from build123d import *

# Parameters (mm, degrees)
SKETCH1_R           = 10
BOSS_EXTRUDE1_DEPTH = 2.5
SKETCH5_W           = 1
SKETCH5_H           = 1
SKETCH6_W           = 1
SKETCH6_H           = 2
BOSS_EXTRUDE2_DEPTH = 0.5
SKETCH7_R           = 0.2
CUT_EXTRUDE1_DEPTH  = 1.5


with BuildPart() as part:
    # Sketch1 → Boss-Extrude1 (new body)
    with BuildSketch(Plane(origin=(0, 0, 0), x_dir=(0, 1, 0), z_dir=(0, 0, 1))):
        with Locations(Location((0, 0, 0), (0, 0, 270))):
            Circle(SKETCH1_R)
    extrude(amount=BOSS_EXTRUDE1_DEPTH)

    # Sketch5 → Cut-Revolve1 (revolve, cut)
    with BuildSketch(Plane(origin=(0, 0, 0), x_dir=(-1, 0, 0), z_dir=(0, 1, 0))):
        with Locations((-4.5, 2)):
            Rectangle(SKETCH5_W, SKETCH5_H)
        with Locations((-2.5, 2)):
            Rectangle(SKETCH5_W, SKETCH5_H)
        with Locations((-6.5, 2)):
            Rectangle(SKETCH5_W, SKETCH5_H)
        with Locations((-8.5, 2)):
            Rectangle(SKETCH5_W, SKETCH5_H)
    revolve(axis=Axis((0, 0, 2.5), (0, 0, -1)), mode=Mode.SUBTRACT)

    # Sketch6 → Boss-Extrude2 (add, symmetric)
    with BuildSketch(Plane(origin=(0, 0, 0), x_dir=(-1, 0, 0), z_dir=(0, 1, 0))):
        with Locations((-2.5, -1)):
            Rectangle(SKETCH6_W, SKETCH6_H)
        with Locations((-4.5, -1)):
            Rectangle(SKETCH6_W, SKETCH6_H)
        with Locations((-6.5, -1)):
            Rectangle(SKETCH6_W, SKETCH6_H)
        with Locations((-8.5, -1)):
            Rectangle(SKETCH6_W, SKETCH6_H)
    extrude(amount=BOSS_EXTRUDE2_DEPTH, both=True)

    # Sketch7 → Cut-Extrude1 (cut, symmetric)
    with BuildSketch(Plane(origin=(0, 0, 0), x_dir=(-1, 0, 0), z_dir=(0, 1, 0))):
        with Locations(Location((-8.5, -1.583373246, 0), (0, 0, 90))):
            Circle(SKETCH7_R)
        with Locations(Location((-6.5, -1.583373246, 0), (0, 0, 90))):
            Circle(SKETCH7_R)
        with Locations(Location((-4.5, -1.583373246, 0), (0, 0, 90))):
            Circle(SKETCH7_R)
        with Locations(Location((-2.5, -1.583373246, 0), (0, 0, 270))):
            Circle(SKETCH7_R)
    extrude(amount=CUT_EXTRUDE1_DEPTH, both=True, mode=Mode.SUBTRACT)


solid = part.part
Here's how the part is built. I have some questions about the finished solid (model axes, mm). A direction names the side the tool comes from. Coordinates: 2 decimals unless noted, no trailing zeros. Loops run counter-clockwise (first coordinate to the right, second up) from the corner with the lowest first, then second, coordinate; pieces in that order, holes last. Notation, with made-up numbers: (-21.5, 4.25) -> (29.5, 4.25) arc R20 cw to (29.5, 20.25) -> close; hole circle Ø7 at (-21, 24). An arc over 180 degrees is marked (long way). Use one line per item in the form item = value. Start each with the question number.
(1) On a 3-axis mill with a long thin cutter (end or side, diameter ignored), from which of +Z, -Z, +X, -X, +Y, -Y can I reach the whole of each face in a straight line? I mean faces 1 (the face through (5, 0, -1)), 2 (the face through (2, 0, -1)), 3 (the face through (2.5, -0.5, -1)). Say none if no direction works.
(2) If we section it at C-C (y = -4.25): Please give me the cut outline in (x, z), then the cut area to 3 significant figures.
(3) Will these pins go through, and if not, where does the flat tip stop? pin 1 (0.8 mm diameter, centred on y = 0, z = -1, fed in from +X); pin 2 (1.1 mm diameter, centred on x = 8.5, z = -1, fed in from +Y); pin 3 (6 mm diameter, centred on x = 4.5, y = 4.5, fed in from -Z).
(4) We'd pull the mould along X, two halves only. Please class faces 4 (the face through (4, 0, -1)), 5 (the face through (4.5, 0.5, -1)), 6 (the face through (9, 0, -1)): pulls with the +X half, pulls with the -X half, needs draft (parallel to the pull), parting line crosses it, or undercut.
(5) Please list where these lines run through material, in increasing order: line 1 along Z through (x, y) = (2.5, -0.15); line 2 along X through (y, z) = (0, -1.3); line 3 along Z through (x, y) = (-8, -1).
(6) If we section it at B-B (x = -5.75): Please give me the cut outline in (y, z).
(7) If we section it at A-A (z = -0.85): Please give me the cut outline in (x, y), then the cut area to 3 significant figures.
(8) If we section it at D-D (z = 0.25): Please give me the cut outline in (x, y), then the cut area to 3 significant figures.
Verdict:
q1.face_1 = -Z, +Y, -Y
q1.face_2 = -Z, -X, +Y, -Y
q1.face_3 = -Z, +X, -X, -Y
q2.outline = (-9.05, 0) -> (9.05, 0) -> (9.05, 2.5) -> (7.93, 2.5) -> (7.93, 1.5) -> (6.78, 1.5) -> (6.78, 2.5) -> (5.56, 2.5) -> (5.56, 1.5) -> (4.24, 1.5) -> (4.24, 2.5) -> (2.63, 2.5) -> (2.63, 1.5) -> (-2.63, 1.5) -> (-2.63, 2.5) -> (-4.24, 2.5) -> (-4.24, 1.5) -> (-5.56, 1.5) -> (-5.56, 2.5) -> (-6.78, 2.5) -> (-6.78, 1.5) -> (-7.93, 1.5) -> (-7.93, 2.5) -> (-9.05, 2.5) -> close
q2.area = 35.0 mm²
q3.pin_1 = 9
q3.pin_2 = 0.5
q3.pin_3 = 0
q4.face_4 = undercut
q4.face_5 = needs draft
q4.face_6 = pulls with the +X half
q5.line_1 = -2 to -1.78, -1.38 to 1.5
q5.line_2 = 2 to 3, 4 to 5, 6 to 7, 8 to 9
q5.line_3 = 0 to 1.5
q6.outline = (-8.18, 0) -> (8.18, 0) -> (8.18, 2.5) -> (6.92, 2.5) -> (6.92, 1.5) -> (5.56, 1.5) -> (5.56, 2.5) -> (3.99, 2.5) -> (3.99, 1.5) -> (1.71, 1.5) -> (1.71, 2.5) -> (-1.71, 2.5) -> (-1.71, 1.5) -> (-3.99, 1.5) -> (-3.99, 2.5) -> (-5.56, 2.5) -> (-5.56, 1.5) -> (-6.92, 1.5) -> (-6.92, 2.5) -> (-8.18, 2.5) -> close
q7.outline = (2, -0.5) -> (3, -0.5) -> (3, 0.5) -> (2, 0.5) -> close; (4, -0.5) -> (5, -0.5) -> (5, 0.5) -> (4, 0.5) -> close; (6, -0.5) -> (7, -0.5) -> (7, 0.5) -> (6, 0.5) -> close; (8, -0.5) -> (9, -0.5) -> (9, 0.5) -> (8, 0.5) -> close
q7.area = 4.00 mm²
q8.outline = circle Ø20 at (0, 0)
q8.area = 314 mm²
